Build history of the part. All positions in model axes, mm. A direction names the side the tool comes from. Round coordinates to 2 decimals unless told otherwise and drop trailing zeros. Write each loop counter-clockwise with the first axis right and the second up, starting at its lowest first coordinate (ties: lowest second). Pieces come first, ordered by that corner, then holes. Notation, with made-up numbers: (-36, -18) -> (-28, -18) arc R6 ccw to (-28, -13) -> close; hole circle Ø1 at (-22.5, -29.5). An arc over 180 degrees is marked (long way). One line per question, with ' | ' between items.
from build123d import *
from OCP.BRepFilletAPI import BRepFilletAPI_MakeChamfer

# Parameters (mm, degrees)
SKETCH1_W            = 76.2
SKETCH1_H            = 38.1
SKETCH1_R            = 2.6035
BOSS_EXTRUDE1_DEPTH  = 6.35
SKETCH4_R            = 2.6035
CUT_EXTRUDE1_DEPTH   = 0.635
SKETCH14_W           = 76.2
SKETCH14_H           = 38.1
SKETCH14_W_2         = 71.12
SKETCH14_H_2         = 33.02
BOSS_EXTRUDE10_DEPTH = 0.635
FILLET6_R            = 3.175
CUT_EXTRUDE4_DEPTH   = 1.27
CUT_EXTRUDE5_DEPTH   = 1.27
CHAMFER1_SIZE        = 1.016
CHAMFER1_SIZE2       = 0.473768581


with BuildPart() as part:
    # Sketch1 → Boss-Extrude1 (new body)
    with BuildSketch(Plane.XY.offset(17.78)):
        with Locations((-38.1, -19.05)):
            Rectangle(SKETCH1_W, SKETCH1_H)
        with Locations((-9.525, -6.731)):
            Circle(SKETCH1_R, mode=Mode.SUBTRACT)
        with Locations((-66.675, -31.75)):
            Circle(SKETCH1_R, mode=Mode.SUBTRACT)
    extrude(amount=BOSS_EXTRUDE1_DEPTH)

    # Sketch4 → Cut-Extrude1 (cut)
    # profile 1 of 2: a face of its own
    with BuildSketch(Plane(origin=(0, 0, 17.78), x_dir=(-1, 0, 0), z_dir=(0, 0, -1))):
        Polygon((0, 0), (0, -13.208), (76.2, -9.017), (76.2, 0), align=None)
        with Locations((9.525, -6.731)):
            Circle(SKETCH4_R, mode=Mode.SUBTRACT)
    # profile 2 of 2: a face of its own
    with BuildSketch(Plane(origin=(0, 0, 17.78), x_dir=(-1, 0, 0), z_dir=(0, 0, -1))):
        Polygon((76.2, -29.083), (0, -24.892), (0, -38.1), (76.2, -38.1), align=None)
        with Locations((66.675, -31.75)):
            Circle(SKETCH4_R, mode=Mode.SUBTRACT)
    extrude(amount=-CUT_EXTRUDE1_DEPTH, mode=Mode.SUBTRACT)

    # Sketch14 → Boss-Extrude10 (add, symmetric)
    with BuildSketch(Plane(origin=(0, 0, 18.415), x_dir=(-1, 0, 0), z_dir=(0, 0, -1))):
        with Locations((38.1, -19.05)):
            Rectangle(SKETCH14_W, SKETCH14_H)
        with Locations((38.1, -19.05)):
            Rectangle(SKETCH14_W_2, SKETCH14_H_2, mode=Mode.SUBTRACT)
    extrude(amount=BOSS_EXTRUDE10_DEPTH, both=True)

    # Fillet6
    fillet6_edges = [part.edges().sort_by_distance(p)[0] for p in [
        (-2.54, -13.0683, 18.0975),
        (-73.66, -9.1567, 18.0975),
        (-73.66, -2.54, 18.0975),
        (-2.54, -2.54, 18.0975),
        (-2.54, -25.0317, 18.0975),
        (-2.54, -35.56, 18.0975),
        (-73.66, -35.56, 18.0975),
        (-73.66, -28.9433, 18.0975),
    ]]
    fillet(fillet6_edges, radius=FILLET6_R)

    # Sketch17 → Cut-Extrude4 (cut)
    with BuildSketch(Plane(origin=(0, 0, 18.415), x_dir=(-1, 0, 0), z_dir=(0, 0, -1))):
        with BuildLine():
            Line((5.715, -2.54), (70.485, -2.54))
            ThreePointArc((70.485, -2.54), (72.73006403, -3.46993597), (73.66, -5.715))
            Line((73.66, -5.715), (73.66, -6.151526439))
            ThreePointArc((73.66, -6.151526439), (72.790886239, -8.334073954), (70.659361477, -9.321735119))
            Line((70.659361477, -9.321735119), (5.889361477, -12.884085119))
            ThreePointArc((5.889361477, -12.884085119), (3.532452485, -12.019762677), (2.54, -9.713876439))
            Line((2.54, -9.713876439), (2.54, -5.715))
            ThreePointArc((2.54, -5.715), (3.46993597, -3.46993597), (5.715, -2.54))
        make_face()
    extrude(amount=-CUT_EXTRUDE4_DEPTH, mode=Mode.SUBTRACT)

    # Sketch20 → Cut-Extrude5 (cut)
    with BuildSketch(Plane(origin=(0, 0, 18.415), x_dir=(-1, 0, 0), z_dir=(0, 0, -1))):
        with BuildLine():
            Line((5.889361477, -25.215914881), (70.659361477, -28.778264881))
            ThreePointArc((70.659361477, -28.778264881), (72.790886239, -29.765926046), (73.66, -31.948473561))
            Line((73.66, -31.948473561), (73.66, -32.385))
            ThreePointArc((73.66, -32.385), (72.73006403, -34.63006403), (70.485, -35.56))
            Line((70.485, -35.56), (5.715, -35.56))
            ThreePointArc((5.715, -35.56), (3.46993597, -34.63006403), (2.54, -32.385))
            Line((2.54, -32.385), (2.54, -28.386123561))
            ThreePointArc((2.54, -28.386123561), (3.532452485, -26.080237323), (5.889361477, -25.215914881))
        make_face()
    extrude(amount=-CUT_EXTRUDE5_DEPTH, mode=Mode.SUBTRACT)

    # Chamfer1: one chamfer whose edges measure the first distance from different faces: ONE call of the kernel's chamfer builder (chamfer() names one face for all edges)
    chamfer1_edges_1 = [part.edges().sort_by_distance(p)[0] for p in [
        (-12.1285, -6.731, 19.685),
    ]]
    chamfer1_side_1 = [part.faces().sort_by_distance(p)[0] for p in [
        (-12.1285, -6.731, 21.9075),
    ]]
    chamfer1_edges_2 = [part.edges().sort_by_distance(p)[0] for p in [
        (-69.2785, -31.75, 19.685),
    ]]
    chamfer1_side_2 = [part.faces().sort_by_distance(p)[0] for p in [
        (-69.2785, -31.75, 21.9075),
    ]]
    chamfer1 = BRepFilletAPI_MakeChamfer(part.part.solid().wrapped)
    for e in chamfer1_edges_1:
        chamfer1.Add(CHAMFER1_SIZE, CHAMFER1_SIZE2, e.wrapped, chamfer1_side_1[0].wrapped)  # the first distance lies on this face
    for e in chamfer1_edges_2:
        chamfer1.Add(CHAMFER1_SIZE, CHAMFER1_SIZE2, e.wrapped, chamfer1_side_2[0].wrapped)  # the first distance lies on this face
    add(Compound.cast(chamfer1.Shape()), mode=Mode.REPLACE)


solid = part.part
(1) Slice it at B-B (x = -5). Write the cut outline in (y, z) (3 decimals), then the cut area to 3 significant figures.
Calculated:
outline: (-38.1, 17.78) -> (-35.478, 17.78) -> (-35.478, 19.685) -> (-25.293, 19.685) -> (-25.293, 17.78) -> (-12.807, 17.78) -> (-12.807, 19.685) -> (-2.622, 19.685) -> (-2.622, 17.78) -> (0, 17.78) -> (0, 24.13) -> (-38.1, 24.13) -> close | area: 203 mm2
(2) Wall check: line 1 (X direction, y = -31.75, z = 23.4); line 2 (Y direction, x = -15, z = 18.5); line 3 (Z direction, x = -16.5, y = -10) (3 decimals). Give the ranges that are in metal, low to high. Write a range as from..to.
Calculated:
line 1: -76.2..-69.28, -64.07..0 | line 2: -38.1..-35.56, -25.72..-12.38, -2.54..0 | line 3: 19.685..24.13
(3) 3-axis set-ups, long thin cutter, end or side, ignore diameter. For faces 1 (the flat face through (-2.54, -8, 19)), 2 (the flat face through (-39, -19, 24.13)): which of +Z, -Z, +X, -X, +Y, -Y reach the whole face in a straight line?
Calculated:
face 1: -Z | face 2: +Z, +X, -X, +Y, -Y
(4) Slice it at C-C (x = -50.5). Write the cut outline in (y, z) (1 decimal), then the cut area to 3 significant figures.
Calculated:
outline: (-38.1, 17.8) -> (-35.6, 17.8) -> (-35.6, 19.7) -> (-27.7, 19.7) -> (-27.7, 17.8) -> (-10.4, 17.8) -> (-10.4, 19.7) -> (-2.5, 19.7) -> (-2.5, 17.8) -> (0, 17.8) -> (0, 24.1) -> (-38.1, 24.1) -> close | area: 212 mm2
(5) Drop flat-ended pins along their axis: pin 1 (3 mm diameter, centred on x = -49, y = -7, fed in from -Z) (3 decimals); pin 2 (3 mm diameter, centred on x = -66.675, y = -31.75, fed in from +Z). Give the stop position or say it passes through.
Calculated:
pin 1: z = 19.685 | pin 2: through
(6) Slice it at A-A (x = -37.5). Write the cut outline in (y, z) (1 decimal), then the cut area to 3 significant figures.
Calculated:
outline: (-38.1, 17.8) -> (-35.6, 17.8) -> (-35.6, 19.7) -> (-27, 19.7) -> (-27, 17.8) -> (-11.1, 17.8) -> (-11.1, 19.7) -> (-2.5, 19.7) -> (-2.5, 17.8) -> (0, 17.8) -> (0, 24.1) -> (-38.1, 24.1) -> close | area: 209 mm2
(7) Mould opens along Y. For faces 3 (the flat face through (-76.2, -19, 21)), 4 (the flat face through (-39, 0, 21)), 5 (the flat face through (-2.54, -30, 19)) say: pulls with the +Y half, pulls with the -Y half, needs draft (parallel to the pull), parting line crosses it, or undercut.
Calculated:
face 3: needs draft | face 4: pulls with the +Y half | face 5: undercut
